Part print with two shaded views. Sizes in mm from the minimum x, y, z corner. Round coordinates to 2 decimals unless told otherwise and drop trailing zeros. Loops run counter-clockwise (first coordinate to the right, second up) from the corner with the lowest first, then second, coordinate; pieces in that order, holes last. Notation, with made-up numbers: (42.25, 52.5) -> (77.25, 52.5) arc R33 ccw to (77.25, 86.5) -> close; hole circle Ø3 at (9.25, 75). An arc over 180 degrees is marked (long way). Use a Markdown table: item, result. Add a question column.
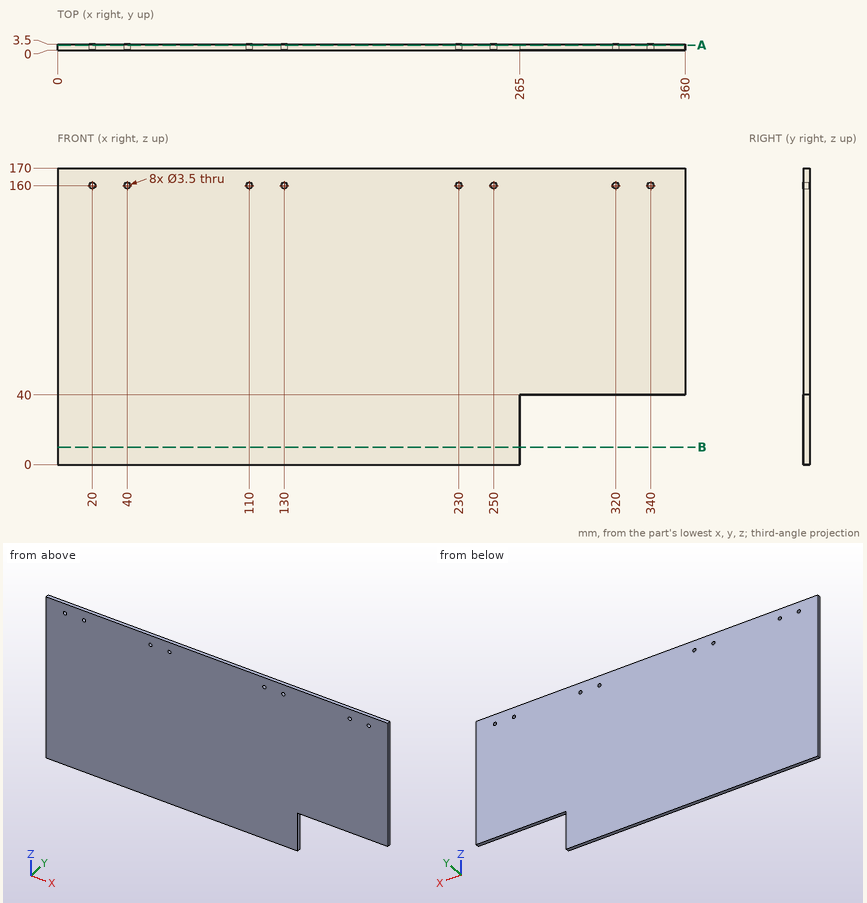
1) Wall check: probe 1 along Z at (x, y) = (249.5, 2.6); probe 2 along Z at (x, y) = (320, 2.35); probe 3 along Z at (x, y) = (325, 2.9). Give the ranges that are in metal, low to high. Write a range as from..to.
2) Pin check, flat tips, straight feed: pin 1 Ø1.5 at (x, z) = (195, 85) entering from -Y; pin 2 Ø1.8 at (x, y) = (323.5, 2.5) entering from -Z. Stop position of each tip, or through.
3) Cut at B-B on z = 10. Write the cut outline in (x, y), and give its area (4 significant figures).
4) Cut at A-A on y = 2.9. Count the separate pieces of the cut face and the enclosed holes in it, and give its area (3 significant figures).
Established:
| question | item | result |
|---|---|---|
| 1 | probe 1 | z = 0..158.32, 161.68..170 |
| 1 | probe 2 | z = 40..158.25, 161.75..170 |
| 1 | probe 3 | z = 40..170 |
| 2 | pin 1 | stops at y = 0 |
| 2 | pin 2 | stops at z = 40 |
| 3 | outline | (0, 0) -> (265, 0) -> (265, 3.5) -> (0, 3.5) -> close |
| 3 | area | 927.5 mm^2 |
| 4 | separate pieces | 1 |
| 4 | enclosed holes | 8 |
| 4 | area | 57,300 mm^2 |
